Read the model definition and answer for the solid it produces. Units are mm, in the model's axes. A direction names the side the tool comes from. Give positions to 0.01 mm unless a question says otherwise; leave off trailing zeros. Order: outer loops, then holes, each group sorted by start corner. A loop starts at its lowest first (then second) coordinate and runs counter-clockwise, first axis right, second up.
Item 1: A cutting plane is placed at B-B (z = 0). Write down the section's boundary in (x, y) (3 decimals).
Item 2: Which of the six approach directions +Z, -Z, +X, -X, +Y, -Y give full straight-line access (tool end or side, diameter ignored) to faces 1 (the face through (8, 3, 0)), 2 (the face through (-2.78, 2, 4)), 3 (the face through (8, -3, 0)), 4 (the face through (-9, -0.5, 4))?
Item 3: A cutting plane is placed at A-A (x = -5.75). Write down the section's boundary in (y, z).
Item 4: Find the intervals of material crossed by line 1 along Y through (x, z) = (-9.5, 0); line 2 along Y through (x, z) = (7.75, 2), in increasing order.
Item 5: A cutting plane is placed at D-D (x = 2.5). Write down the section's boundary in (y, z) (3 decimals), plus the area to 3 significant figures.
Item 6: A cutting plane is placed at C-C (y = -2). Write down the section's boundary in (x, z), plus the area to 3 significant figures.
Item 7: The mould has two halves that part along Z. Classify faces 5 (the face through (-9, 0.5, -4)), 6 (the face through (8, 0, 3)), 7 (the face through (-2.78, 0, 0)), 8 (the face through (-8.357, -1.092, 2.633)): +Z half, -Z half, draft (parallel to the pull), parting line (faces both ways), or undercut.
Item 8: Given pin 1 Ø3 at (x, z) = (11, -1.5) entering from -Y; pin 2 Ø2 at (x, z) = (-5.5, -1) entering from +Y; pin 3 Ø3.5 at (y, z) = (0, 0) entering from -X, each flat-ended and moving along its own axis, determine where each tip first touches the part or whether it passes through.
from build123d import *

# Parameters (mm, degrees)
SKETCH1_R           = 4.765
BOSS_EXTRUDE1_DEPTH = 2.78
SKETCH2_R           = 4.25
BOSS_EXTRUDE2_DEPTH = 11
SKETCH3_W           = 6
SKETCH3_H           = 6
BOSS_EXTRUDE3_DEPTH = 11
CUT_EXTRUDE1_START  = 11
SKETCH4_R           = 2.85
CUT_EXTRUDE1_DEPTH  = 11
CUT_EXTRUDE2_START  = -10
CUT_EXTRUDE2_DEPTH  = 10


with BuildPart() as part:
    # Sketch1 → Boss-Extrude1 (new, symmetric)
    with BuildSketch(Plane(origin=(0, 0, 0), x_dir=(0, 0, -1), z_dir=(1, 0, 0))):
        Circle(SKETCH1_R)
    extrude(amount=BOSS_EXTRUDE1_DEPTH, both=True)

    # Sketch2 → Boss-Extrude2 (add)
    with BuildSketch(Plane.ZY.offset(2.78)):
        Circle(SKETCH2_R)
    extrude(amount=BOSS_EXTRUDE2_DEPTH)

    # Sketch3 → Boss-Extrude3 (add)
    with BuildSketch(Plane(origin=(2.78, 0, 0), x_dir=(0, 0, -1), z_dir=(1, 0, 0))):
        Rectangle(SKETCH3_W, SKETCH3_H)
    extrude(amount=BOSS_EXTRUDE3_DEPTH)

    # Sketch4 → Cut-Extrude1 (cut)
    with BuildSketch(Plane.ZY.offset(2.78).offset(CUT_EXTRUDE1_START)):
        Circle(SKETCH4_R)
    extrude(amount=-CUT_EXTRUDE1_DEPTH, mode=Mode.SUBTRACT)

    # Sketch5 → Cut-Extrude2 (cut)
    with BuildSketch(Plane.ZY.offset(13.78).offset(CUT_EXTRUDE2_START)):
        with BuildLine():
            ThreePointArc((-4.220485754, 0.5), (-4.25, 0), (-4.220485754, -0.5))
            Line((-4.220485754, -0.5), (-2.805797569, -0.5))
            ThreePointArc((-2.805797569, -0.5), (-2.85, 0), (-2.805797569, 0.5))
            Line((-2.805797569, 0.5), (-4.220485754, 0.5))
        make_face()
        with BuildLine():
            Line((2.805797569, -0.5), (4.220485754, -0.5))
            ThreePointArc((4.220485754, -0.5), (4.242615022, -0.250435167), (4.25, 0))
            ThreePointArc((4.25, 0), (4.242615022, 0.250435167), (4.220485754, 0.5))
            Line((4.220485754, 0.5), (2.805797569, 0.5))
            ThreePointArc((2.805797569, 0.5), (2.838927885, 0.250975026), (2.85, 0))
            ThreePointArc((2.85, 0), (2.838927885, -0.250975026), (2.805797569, -0.5))
        make_face()
        with BuildLine():
            ThreePointArc((-4.73869444, 0.5), (-4.765, 0), (-4.73869444, -0.5))
            Line((-4.73869444, -0.5), (-4.220485754, -0.5))
            ThreePointArc((-4.220485754, -0.5), (-4.25, 0), (-4.220485754, 0.5))
            Line((-4.220485754, 0.5), (-4.73869444, 0.5))
        make_face()
        with BuildLine():
            ThreePointArc((-2.805797569, 0.5), (-2.85, 0), (-2.805797569, -0.5))
            Line((-2.805797569, -0.5), (2.805797569, -0.5))
            ThreePointArc((2.805797569, -0.5), (2.838927885, -0.250975026), (2.85, 0))
            ThreePointArc((2.85, 0), (2.838927885, 0.250975026), (2.805797569, 0.5))
            Line((2.805797569, 0.5), (-2.805797569, 0.5))
        make_face()
        with BuildLine():
            ThreePointArc((4.25, 0), (4.242615022, -0.250435167), (4.220485754, -0.5))
            Line((4.220485754, -0.5), (4.73869444, -0.5))
            ThreePointArc((4.73869444, -0.5), (4.765, 0), (4.73869444, 0.5))
            Line((4.73869444, 0.5), (4.220485754, 0.5))
            ThreePointArc((4.220485754, 0.5), (4.242615022, 0.250435167), (4.25, 0))
        make_face()
    extrude(amount=CUT_EXTRUDE2_DEPTH, mode=Mode.SUBTRACT)


solid = part.part
Response values:
1. outline: (-13.78, -4.25) - (-2.78, -4.25) - (-2.78, -4.765) - (2.78, -4.765) - (2.78, -3) - (13.78, -3) - (13.78, 3) - (2.78, 3) - (2.78, 4.765) - (-2.78, 4.765) - (-2.78, 4.25) - (-13.78, 4.25) - (-13.78, 2.85) - (-2.78, 2.85) - (-2.78, -2.85) - (-13.78, -2.85) - close
2. face 1: +Z, -Z, +X, +Y
2. face 2: -X
2. face 3: +Z, -Z, +X, -Y
2. face 4: +Z, -Z, -X
3. outline: (-0.5, -4.22) - (-0.5, -2.81) arc R2.85 cw to (-0.5, 2.81) - (-0.5, 4.22) arc R4.25 ccw to start; (0.5, -4.22) arc R4.25 ccw to (0.5, 4.22) - (0.5, 2.81) arc R2.85 cw to (0.5, -2.81) - close
4. line 1: y = -4.25 to -2.85, 2.85 to 4.25
4. line 2: y = -3 to 3
5. outline: circle Ø9.53 at (0, 0)
5. area: 71.3 mm2
6. outline: (-13.78, -3.75) - (-2.78, -3.75) - (-2.78, -4.32) - (2.78, -4.32) - (2.78, -3) - (13.78, -3) - (13.78, 3) - (2.78, 3) - (2.78, 4.32) - (-2.78, 4.32) - (-2.78, 3.75) - (-13.78, 3.75) - (-13.78, 2.03) - (-2.78, 2.03) - (-2.78, -2.03) - (-13.78, -2.03) - close
6. area: 152 mm2
7. face 5: draft
7. face 6: +Z half
7. face 7: undercut
7. face 8: undercut
8. pin 1: stops at y = -3
8. pin 2: stops at y = 4.25
8. pin 3: stops at x = -2.78
